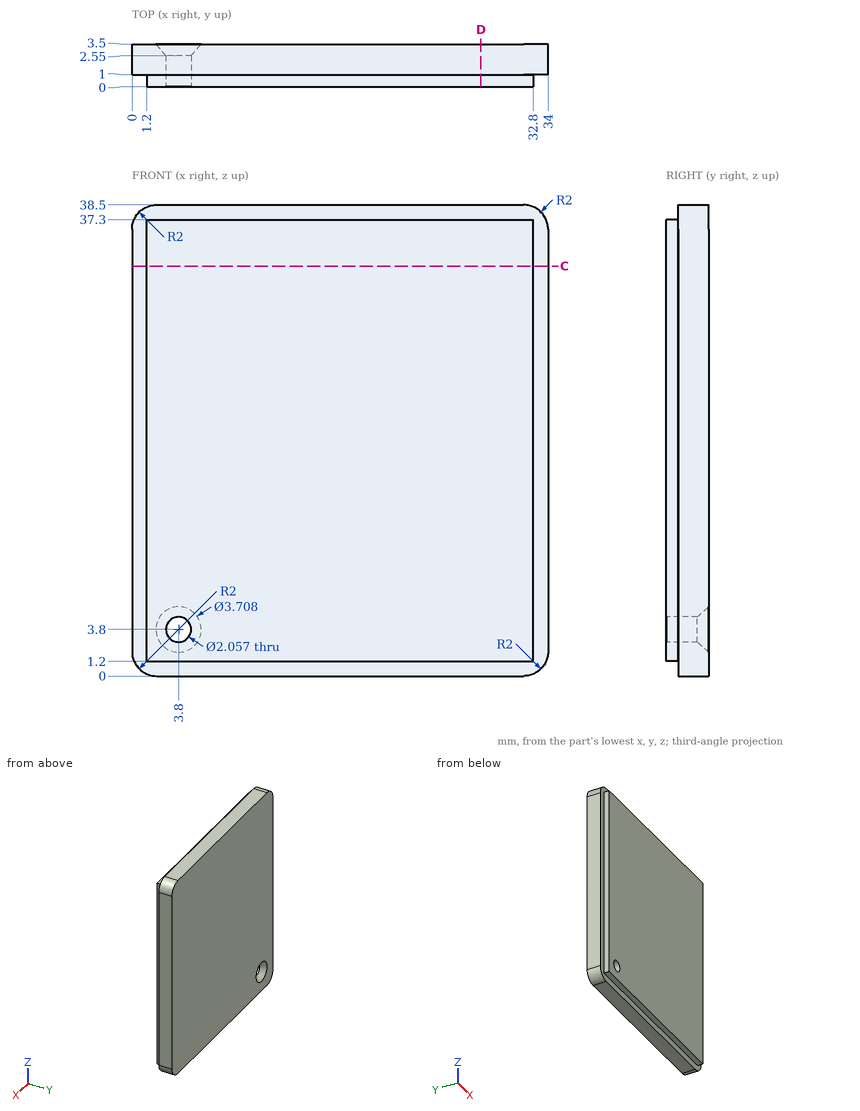
Geometry check sheet. Reference: drawing and pictorial views, mm from the part's lowest x, y, z. Give positions to 0.01 mm unless a question says otherwise; leave off trailing zeros. Loops run counter-clockwise (first coordinate to the right, second up) from the corner with the lowest first, then second, coordinate; pieces in that order, holes last. Notation, with made-up numbers: (-16, -27.5) - (32, -27.5) arc R31 ccw to (32, 7.5) - close; hole circle Ø4 at (-20, 43.25). An arc over 180 degrees is marked (long way). One line per question, with ' | ' between items. Start each with the question number.
1. Gauge pin test, flat ends, axial feed: pin 1 Ø8 at (x, z) = (13.5, 24.5) entering from -Y; pin 2 Ø0.5 at (x, y) = (13, 0.5) entering from -Z; pin 3 Ø0.5 at (y, z) = (0.5, 24) entering from +X. Record the tip position at first contact, or that the pin passes through.
2. Material ranges on line 1 along X through (y, z) = (1.55, 3.8); line 2 along X through (y, z) = (0.95, 23.5); line 3 along Z through (x, y) = (22, 0.4), recorded low to high. Write a range as [from, to].
3. Cross-section at D-D, the plane x = 28.5. Enter the section's corners in (y, z), plus the area to 3 significant figures.
4. Cross-section at C-C, the plane z = 33.5. Enter the section's corners in (x, y), plus the area to 3 significant figures.
Check result:
1) pin 1: stops at y = 0 | pin 2: stops at z = 1.2 | pin 3: stops at x = 32.8
2) line 1: x = [0, 2.77], [4.83, 34] | line 2: x = [1.2, 32.8] | line 3: z = [1.2, 37.3]
3) outline: (0, 1.2) - (1, 1.2) - (1, 0) - (3.5, 0) - (3.5, 38.5) - (1, 38.5) - (1, 37.3) - (0, 37.3) - close | area: 132 mm2
4) outline: (0, 1) - (1.2, 1) - (1.2, 0) - (32.8, 0) - (32.8, 1) - (34, 1) - (34, 3.5) - (0, 3.5) - close | area: 117 mm2
